CAD build for the part. Positions are in the model's coordinates, mm. Face numbers are marked on the shaded views. A direction names the side the tool comes from. Give positions to 0.01 mm unless a question says otherwise; leave off trailing zeros. Loops run counter-clockwise (first coordinate to the right, second up) from the corner with the lowest first, then second, coordinate; pieces in that order, holes last. Notation, with made-up numbers: M 87,-27.75 L 112,-27.75 A25 cw 112,-5.75 Z; hole C -10,44.5 d2. An arc over 180 degrees is marked long. One line per question, with ' | ' between items.
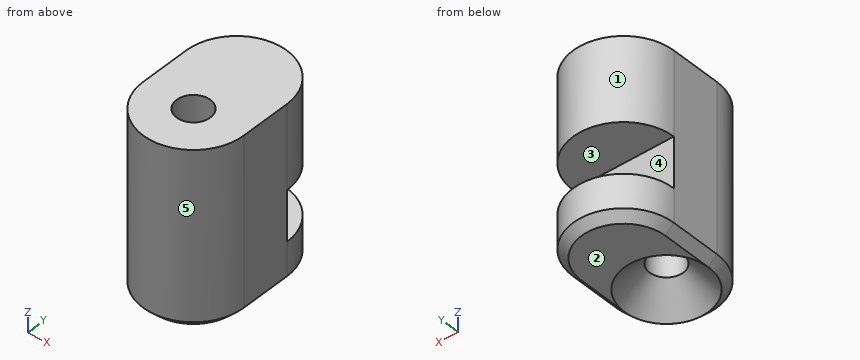
Autodesk Inventor part; units mm, degrees
ref_plane "YZ Plane" through (0, 0, 0) normal (1, 0, 0) x (0, 1, 0)
ref_plane "XZ Plane" through (0, 0, 0) normal (0, 1, 0) x (-1, 0, 0)
ref_plane "XY Plane" through (0, 0, 0) normal (0, 0, 1) x (1, 0, 0)
sketch "Sketch2" plane through (0, 0, 0) normal (0, 0, 1) x (1, 0, 0)
  circle A0 centre (0, 0) radius 6
  circle A1 centre (0, 0) radius 2
  dimension "d0" = 12
  dimension "d1" = 4
extrude "Extrusion1" add sketch "Sketch2" along normal blind 21
sketch "Sketch3" plane through (0, 0, 21) normal (0, 0, 1) x (1, 0, 0)
  line L0 (0, 0) -> (0, 6) construction
  line L1 (6, 0) -> (6, 6)
  line L2 (-6, 6) -> (-6, 0)
  arc A0 (-6, 0) -> (6, 0) centre (0, 0) ccw
  arc A1 (6, 6) -> (-6, 6) centre (0, 6) ccw
  circle A2 centre (0, 0) radius 2
  circle A3 centre (0, 0) radius 6
  circle A4 centre (0, 0) radius 2
  circle A5 centre (0, 0) radius 6
  point P0 (0, 3)
  dimension "d4" = 6
  dimension "d5" = 6
extrude "Extrusion2" add sketch "Sketch3" against normal blind 10 contours A3 L2 A1 L1
sketch "Sketch4" plane through (0, 0, 0) normal (0, 0, -1) x (-1, 0, 0)
  arc A0 (6, 6) -> (-6, 6) centre (0, 6) ccw
  line L0 (-6, 6) -> (-6, 0)
  line L1 (6, 0) -> (6, 6)
  arc A1 (6, 0) -> (-6, 0) centre (0, 0) ccw
  circle A2 centre (0, 0) radius 2
extrude "Extrusion3" add sketch "Sketch4" against normal blind 5 contours L1 A1 L0 A0
sketch "Sketch5" plane through (0, 0, 11) normal (0, 0, -1) x (-1, 0, 0)
  arc A0 (6, 6) -> (-6, 6) centre (0, 6) ccw
  line L0 (-6, 6) -> (-6, 0)
  line L1 (6, 0) -> (6, 6)
  arc A1 (6, 0) -> (-6, 0) centre (0, 0) ccw
  line L2 (-6, 6) -> (6, 6)
  arc A2 (6, 0) -> (-6, 0) centre (0, 0) ccw
  point P0 (0, 6)
extrude "Extrusion4" add sketch "Sketch5" along normal blind 6.4 contours L1 A1 L2 | L2 A1 L0
chamfer "Chamfer1" distance 3 angle 45 1 edges at (-2, 0, 0)
chamfer "Chamfer2" distance 1 angle 45 4 edges at (-6, 3, 0) (0, 12, 0) (6, 3, 0) (0, -6, 0)
properties part number "picture-fixings-6mm"
Item 1: Saw through at C-C on z = 8.25. Give the cut face in (x, y), and give its area (3 significant figures).
Conclusion:
outline: M -6,0 A6 ccw 6,0 L 6,6 L -6,6 Z; hole C 0,0 d4 | area: 116 mm²
Item 2: Mould opens along Z. For the marked faces 1, 2 and 3 say: pulls with the +Z half, pulls with the -Z half, needs draft (parallel to the pull), parting line crosses it, or undercut.
Conclusion:
face 1: needs draft | face 2: pulls with the -Z half | face 3: undercut
Item 3: Saw through at B-B on z = 13. Give the cut face in (x, y).
Conclusion:
outline: M -6,0 A6 ccw 6,0 L 6,6 A6 ccw -6,6 Z; hole C 0,0 d4
Item 4: Drop flat-ended pins along their axis: P1, Ø2.5, axis at x = 0, y = 0, coming from the -Z side; P2, Ø2, axis at x = -3.5, z = 12.5, coming from the -Y side; P3, Ø1.5, axis at x = 3.5, z = 6.5, coming from the -Y side; P4, Ø3, axis at x = -0.5, y = -1, coming from the -Z side. Give the stop position or say it passes through.
Conclusion:
P1: through | P2: y = -5.45 | P3: y = -5.33 | P4: z = 2.38
Item 5: Drill centre lines: line 1 along Z through (x, y) = (-3.75, 9); line 2 along Y through (x, z) = (0, 15.25); line 3 along Y through (x, z) = (0, 10). Where is each one in solid material? Low to high. Write a range as [from, to].
Conclusion:
line 1: [0, 5], [11, 21] | line 2: [-6, -2], [2, 12] | line 3: [-6, -2], [2, 6]
Item 6: 3-axis set-ups, long thin cutter, end or side, ignore diameter. For the marked faces 4 and 5: which of +Z, -Z, +X, -X, +Y, -Y reach the whole face in a straight line?
Conclusion:
face 4: +X, -X, +Y | face 5: +Z, -Z, -Y
